The listing builds one solid part. Answer for the finished solid, in the listing's coordinates (mm). Face numbers are marked on the shaded views. A direction names the side the tool comes from. Give positions to 0.01 mm unless a question says otherwise; leave off trailing zeros. Order: outer loops, then holes, each group sorted by start corner. A loop starts at its lowest first (then second) coordinate and runs counter-clockwise, first axis right, second up. Notation, with made-up numbers: (81.25, 61) -> (124.25, 61) arc R18 cw to (124.25, 71) -> close; hole circle Ø6 at (33.5, 8.5). An arc over 180 degrees is marked (long way). Write item = value, one per line. Start each with the question number.
```python
from build123d import *

# Parameters (mm, degrees)
SKETCH003_R  = 6
PAD001_DEPTH = 22.5
SKETCH001_R  = 6
PAD_DEPTH    = 22.5


with BuildPart() as pad001:
    # Sketch003 → Pad001 (new body, symmetric)
    with BuildSketch(Plane.YZ):
        with Locations((0, 73)):
            Circle(SKETCH003_R)
    extrude(amount=PAD001_DEPTH, both=True)


with BuildPart() as pad:
    # Sketch001 → Pad (new body, symmetric)
    with BuildSketch(Plane.XZ):
        with Locations((0, 73)):
            Circle(SKETCH001_R)
    extrude(amount=PAD_DEPTH, both=True)


with BuildPart() as cut001:
    # Sketch → Revolution (revolve)
    with BuildSketch(Plane.XZ):
        with BuildLine():
            Line((0, 65.425804), (4.000562, 65.425804))
            Line((4.000562, 65.425804), (11.168226, 68.592918))
            Line((11.168226, 68.592918), (6.667604, 56.924622))
            Line((6.667604, 56.924622), (10.834842, 56.924622))
            Line((10.834842, 56.924622), (10.834842, 53.424126))
            Line((10.834842, 53.424126), (8.337257, 53.424126))
            Line((8.337257, 53.424126), (8.337257, 26.713955))
            Line((8.337257, 26.713955), (19.875788, 4.581964))
            ThreePointArc((17.097317, 0), (19.776603, 1.508704), (19.875788, 4.581964))
            Line((0, 0), (17.097317, 0))
            Line((0, 65.425804), (0, 0))
        make_face()
    revolve(axis=Axis((0, 0, 0), (0, 0, 1)))

    # Cut: cut Pad
    add(pad.part, mode=Mode.SUBTRACT)

    # Cut001: cut Pad001
    add(pad001.part, mode=Mode.SUBTRACT)


solid = cut001.part
```
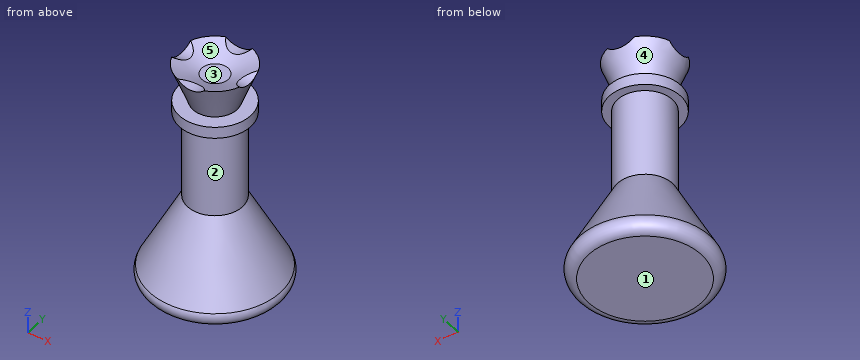
Item 1: Consider L1, parallel to Z at x = 3.5, y = -2; L2, parallel to Z at x = 6.5, y = 12; L3, parallel to Y at x = -2, z = 57. Determine where each line is inside the solid, lowest interval first. Write a range as from..to.
Item 2: A cutting plane is placed at D-D, the plane z = 60.5. Write down the section's boundary in (x, y).
Item 3: Flat-ended cylindrical pins translate along their axes: pin 1 (5 mm diameter, centred on y = 0, z = 42, fed in from -X); pin 2 (9 mm diameter, centred on x = -2, y = -1, fed in from +Z); pin 3 (3 mm diameter, centred on x = 2.5, z = 57, fed in from +Y). Find the tip coordinate at first contact, or state that the pin passes through.
Item 4: The mould has two halves that part along Z. Classify the marked faces 1, 2 and 3: +Z half, -Z half, draft (parallel to the pull), parting line (faces both ways), or undercut.
Item 5: A cutting plane is placed at A-A, the plane x = 0. Write down the section's boundary in (y, z), plus the area to 3 significant figures.
Item 6: A cutting plane is placed at C-C, the plane z = 49. Write down the section's boundary in (x, y).
Item 7: Which of the six approach directions +Z, -Z, +X, -X, +Y, -Y give full straight-line access (tool end or side, diameter ignored) to the marked faces 4 and 5?
Check values:
q1.L1 = 0..65.44
q1.L2 = 0..16.53
q1.L3 = -6.39..6.39
q2.outline = circle Ø16.09 at (0, 0)
q3.pin_1 = -8.34
q3.pin_2 = 66.63
q3.pin_3 = 10.79
q4.face_1 = -Z half
q4.face_2 = undercut
q4.face_3 = +Z half
q5.outline = (-19.88, 4.58) arc R3.13 ccw to (-17.1, 0) -> (17.1, 0) arc R3.13 ccw to (19.88, 4.58) -> (8.34, 26.71) -> (8.34, 53.42) -> (10.83, 53.42) -> (10.83, 56.92) -> (6.67, 56.92) -> (10.55, 67) -> (7.56, 67) -> (4, 65.43) -> (-4, 65.43) -> (-7.56, 67) -> (-10.55, 67) -> (-6.67, 56.92) -> (-10.83, 56.92) -> (-10.83, 53.42) -> (-8.34, 53.42) -> (-8.34, 26.71) -> close
q5.area = 1,480 mm^2
q6.outline = circle Ø16.67 at (0, 0)
q7.face_4 = none
q7.face_5 = +Z
